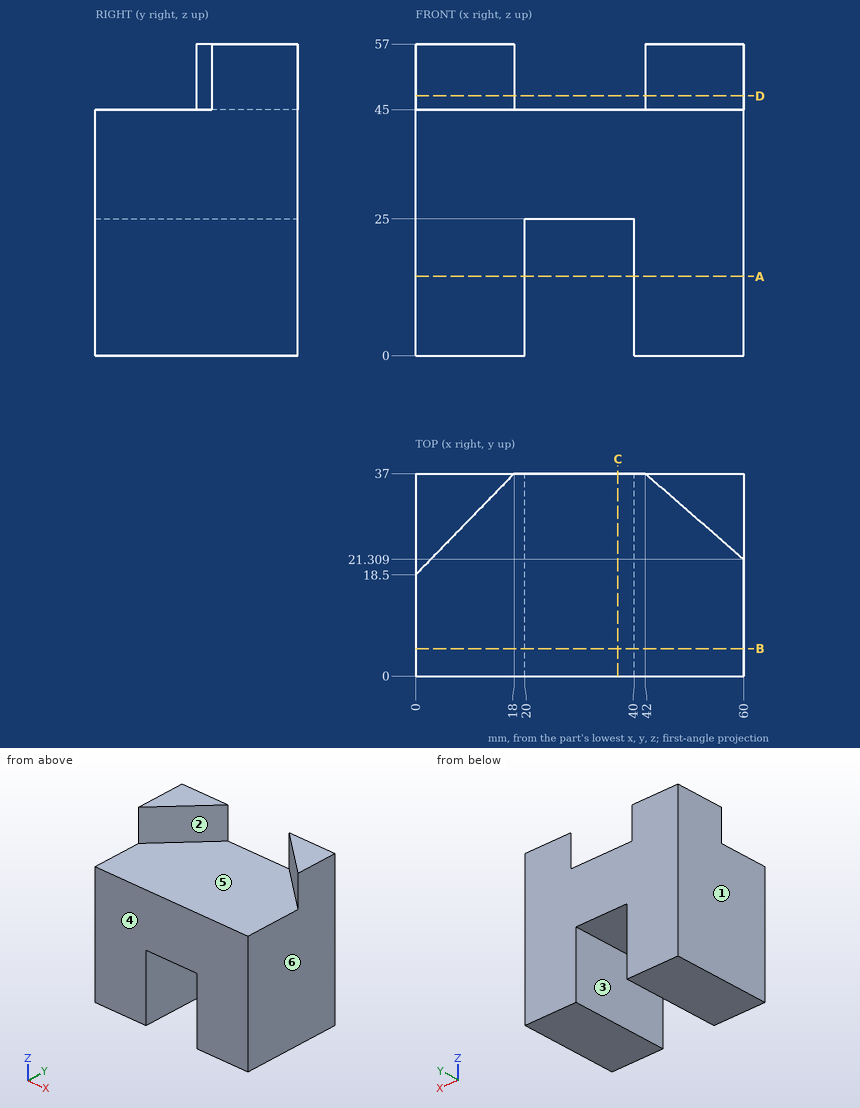
Source: three-view drawing plus pictorial views. Frame: mm from the lowest corner of the part. A direction names the side the tool comes from. Round coordinates to 2 decimals unless told otherwise and drop trailing zeros. Loops run counter-clockwise (first coordinate to the right, second up) from the corner with the lowest first, then second, coordinate; pieces in that order, holes last.
Q1. Access query for the marked faces 1, 2 and 3. Directions: +Z, -Z, +X, -X, +Y, -Y. A direction counts if a zero-diameter tool reaches every point of the face in a straight line with its end or side. Return the directions, or none.
Q2. Section D-D on z = 47.5. Return loops of the section in (x, y).
Q3. Material intervals for L1, parallel to X at y = 22, z = 2; L2, parallel to Z at x = 17, y = 31; L3, parallel to Z at x = 31.5, y = 6, sorted ascending.
Q4. Section C-C on x = 37. Return loops of the section in (y, z), plus the area to 3 significant figures.
Q5. Section B-B on y = 5. Return loops of the section in (x, z).
Q6. Pull-direction query (X, two-part tool) for the marked faces 4, 5 and 6; classes: released by +X, released by -X, zero draft, split by the parting line, or undercut.
Q7. Pin query (flat end, axial travel): P1, Ø10, axis at x = 27.5, y = 17, coming from the -Z side. Return the tip coordinate at first contact, or that it passes through.
Q8. Section A-A on z = 14.5. Return loops of the section in (x, y), plus the area to 3 significant figures.
Evaluation:
1. face 1: +Z, -Z, -X, +Y, -Y
1. face 2: +Z, -Y
1. face 3: -Z, +Y, -Y
2. outline: (0, 18.5) - (18, 37) - (0, 37) - close; (42, 37) - (60, 21.31) - (60, 37) - close
3. L1: x = 0 to 20, 40 to 60
3. L2: z = 0 to 45
3. L3: z = 25 to 45
4. outline: (0, 25) - (37, 25) - (37, 45) - (0, 45) - close
4. area: 740 mm2
5. outline: (0, 0) - (20, 0) - (20, 25) - (40, 25) - (40, 0) - (60, 0) - (60, 45) - (0, 45) - close
6. face 4: zero draft
6. face 5: undercut
6. face 6: released by +X
7. P1: stops at z = 25
8. outline: (0, 0) - (20, 0) - (20, 37) - (0, 37) - close; (40, 0) - (60, 0) - (60, 37) - (40, 37) - close
8. area: 1,480 mm2
